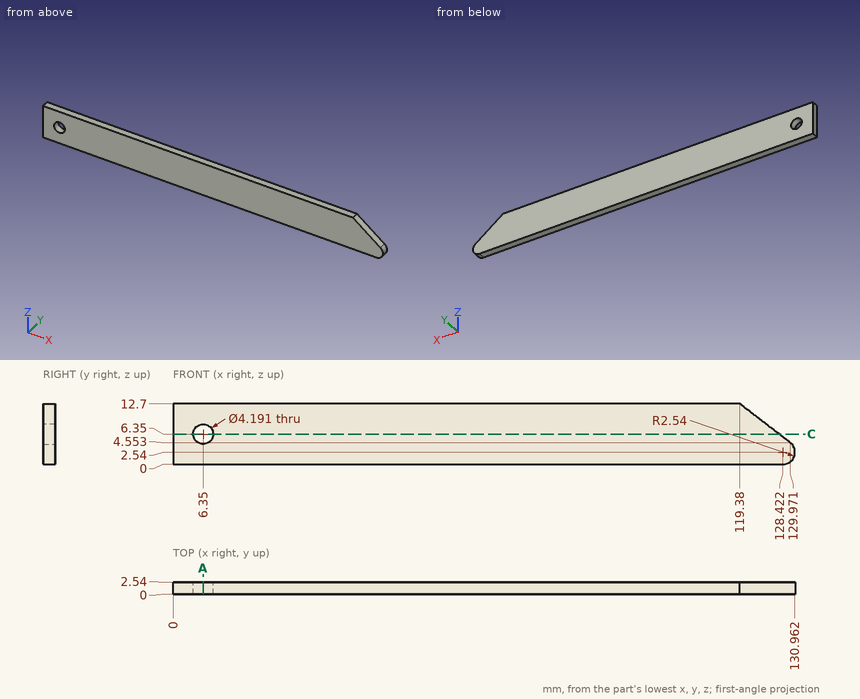
Verification items for this drawing (mm, ordinates from the low corner). Coordinates: 2 decimals unless noted, no trailing zeros. Order: outer loops, then holes, each group sorted by start corner. A loop starts at its lowest first (then second) coordinate and runs counter-clockwise, first axis right, second up. Notation, with made-up numbers: (48.25, -7.5) - (86.25, -7.5) arc R9 cw to (86.25, 8.5) - close; hole circle Ø11 at (1, 26.5). An arc over 180 degrees is marked (long way). Answer in a Markdown table with one row per item. Add a question column.
1. Material ranges on L1, parallel to X at y = 0.15, z = 6.75 (1 decimal); L2, parallel to X at y = 2, z = 6.35 (1 decimal); L3, parallel to X at y = 1.65, z = 2.75, recorded low to high. Write a range as [from, to].
2. Section check C-C (z = 6.35). Enter the section's corners in (x, y) (1 decimal).
3. Section check A-A (x = 6.35). Enter the section's corners in (y, z) (1 decimal), plus the area to 3 significant figures.
Data:
| question | item | result |
|---|---|---|
| 1 | L1 | x = [0, 4.3], [8.4, 127.1] |
| 1 | L2 | x = [0, 4.3], [8.4, 127.6] |
| 1 | L3 | x = [0, 130.95] |
| 2 | outline | (0, 0) - (4.3, 0) - (4.3, 2.5) - (0, 2.5) - close; (8.4, 0) - (127.6, 0) - (127.6, 2.5) - (8.4, 2.5) - close |
| 3 | outline | (0, 0) - (2.5, 0) - (2.5, 4.3) - (0, 4.3) - close; (0, 8.4) - (2.5, 8.4) - (2.5, 12.7) - (0, 12.7) - close |
| 3 | area | 21.6 mm² |
